For this review, take the finished solid that the model builds, in its own axes (mm). Round coordinates to 2 decimals unless told otherwise and drop trailing zeros. Order: outer loops, then holes, each group sorted by start corner. A loop starts at its lowest first (then second) coordinate and runs counter-clockwise, first axis right, second up. Notation, with made-up numbers: M -31,-33.75 L 20,-33.75 A4 ccw 20,-29.75 Z; hole C 15,-30 d8. An arc over 180 degrees is marked long. Use a Markdown table: item, result.
from build123d import *

# Parameters (mm, degrees)
BOSS_EXTRUDE1_DEPTH = 5
CHAMFER1_SIZE       = 3
SKETCH4_W           = 10
SKETCH4_H           = 2
BOSS_EXTRUDE3_DEPTH = 2
SKETCH5_W           = 2
SKETCH5_H           = 10
BOSS_EXTRUDE4_DEPTH = 12
CHAMFER2_SIZE       = 2
SKETCH6_W           = 10
SKETCH6_H           = 2
BOSS_EXTRUDE5_DEPTH = 1
CHAMFER3_SIZE       = 1
SKETCH7_W           = 10
SKETCH7_H           = 2
BOSS_EXTRUDE6_DEPTH = 2
SKETCH8_W           = 2
SKETCH8_H           = 10
BOSS_EXTRUDE7_DEPTH = 12
CHAMFER4_SIZE       = 2
SKETCH9_W           = 10
SKETCH9_H           = 2
BOSS_EXTRUDE8_DEPTH = 1
CHAMFER5_SIZE       = 1


with BuildPart() as part:
    # Sketch1 → Boss-Extrude1 (new body)
    with BuildSketch(Plane(origin=(0, 0, 0), x_dir=(1, 0, 0), z_dir=(0, 1, 0))):
        Polygon((-96.805555556, 26.527777778), (-46.805555556, 26.527777778), (-46.805555556, 76.527777778), (57.194444444, 76.527777778), (57.194444444, 26.527777778), (107.194444444, 26.527777778), (107.194444444, -43.472222222), (-96.805555556, -43.472222222), align=None)
    extrude(amount=BOSS_EXTRUDE1_DEPTH)

    # Chamfer1
    chamfer1_edges = [part.edges().sort_by_distance(p)[0] for p in [
        (107.194444444, 5, 8.472222222),
        (82.194444444, 5, -26.527777778),
        (57.194444444, 5, -51.527777778),
        (5.194444444, 5, -76.527777778),
        (-46.805555556, 5, -51.527777778),
        (-71.805555556, 5, -26.527777778),
        (-96.805555556, 5, 8.472222222),
        (5.194444444, 5, 43.472222222),
    ]]
    chamfer(chamfer1_edges, length=CHAMFER1_SIZE)

    # Sketch4 → Boss-Extrude3 (add)
    with BuildSketch(Plane(origin=(107.194444444, 0, 0), x_dir=(0, 0, -1), z_dir=(1, 0, 0))):
        with Locations((-8.472222222, 1)):
            Rectangle(SKETCH4_W, SKETCH4_H)
    extrude(amount=BOSS_EXTRUDE3_DEPTH)

    # Sketch5 → Boss-Extrude4 (add)
    with BuildSketch(Plane(origin=(0, 2, 0), x_dir=(1, 0, 0), z_dir=(0, 1, 0))):
        with Locations((108.194444444, -8.472222222)):
            Rectangle(SKETCH5_W, SKETCH5_H)
    extrude(amount=BOSS_EXTRUDE4_DEPTH)

    # Chamfer2
    chamfer2_edges = [part.edges().sort_by_distance(p)[0] for p in [
        (107.194444444, 14, 8.472222222),
    ]]
    chamfer(chamfer2_edges, length=CHAMFER2_SIZE - 0.0001)  # a hair under: the kernel refuses the full size

    # Sketch6 → Boss-Extrude5 (add)
    with BuildSketch(Plane.ZY.offset(-107.194444444)):
        with Locations((8.472222222, 11)):
            Rectangle(SKETCH6_W, SKETCH6_H)
    extrude(amount=BOSS_EXTRUDE5_DEPTH)

    # Chamfer3
    chamfer3_edges = [part.edges().sort_by_distance(p)[0] for p in [
        (106.194444444, 10, 8.472222222),
        (106.194444444, 12, 8.472222222),
    ]]
    chamfer(chamfer3_edges, length=CHAMFER3_SIZE - 0.0001)  # a hair under: the kernel refuses the full size

    # Sketch7 → Boss-Extrude6 (add)
    with BuildSketch(Plane.ZY.offset(96.805555556)):
        with Locations((8.472222222, 1)):
            Rectangle(SKETCH7_W, SKETCH7_H)
    extrude(amount=BOSS_EXTRUDE6_DEPTH)

    # Sketch8 → Boss-Extrude7 (add)
    with BuildSketch(Plane(origin=(0, 2, 0), x_dir=(1, 0, 0), z_dir=(0, 1, 0))):
        with Locations((-97.805555556, -8.472222222)):
            Rectangle(SKETCH8_W, SKETCH8_H)
    extrude(amount=BOSS_EXTRUDE7_DEPTH)

    # Chamfer4
    chamfer4_edges = [part.edges().sort_by_distance(p)[0] for p in [
        (-96.805555556, 14, 8.472222222),
    ]]
    chamfer(chamfer4_edges, length=CHAMFER4_SIZE - 0.0001)  # a hair under: the kernel refuses the full size

    # Sketch9 → Boss-Extrude8 (add)
    with BuildSketch(Plane(origin=(-96.805555556, 0, 0), x_dir=(0, 0, -1), z_dir=(1, 0, 0))):
        with Locations((-8.472222222, 11)):
            Rectangle(SKETCH9_W, SKETCH9_H)
    extrude(amount=BOSS_EXTRUDE8_DEPTH)

    # Chamfer5
    chamfer5_edges = [part.edges().sort_by_distance(p)[0] for p in [
        (-95.805555556, 10, 8.472222222),
        (-95.805555556, 12, 8.472222222),
    ]]
    chamfer(chamfer5_edges, length=CHAMFER5_SIZE - 0.0001)  # a hair under: the kernel refuses the full size


solid = part.part
Q1. Add section A-A (x = -7). Write out the cut boundary in (y, z).
Determined:
| item | result |
|---|---|
| outline | M 0,-76.53 L 2,-76.53 L 5,-73.53 L 5,40.47 L 2,43.47 L 0,43.47 Z |
Q2. Clearance check with flat-ended pins moving along their axes: pin 1 (1.6 mm diameter, centred on y = 0.5, z = 29, fed in from +X); pin 2 (0.9 mm diameter, centred on x = -97, y = 5, fed in from -Z); pin 3 (0.9 mm diameter, centred on x = 107, y = 6.5, fed in from +Z). State where each tip first meets the part, or that it passes through.
Determined:
| item | result |
|---|---|
| pin 1 | stops at x = 107.19 |
| pin 2 | stops at z = 3.47 |
| pin 3 | stops at z = 13.47 |
Q3. Wall thickness on line 1 along X through (y, z) = (6, 4.5); line 2 along Y through (x, z) = (4.5, -35); line 3 along X through (y, z) = (4, 10): over which ranges is each line inside the solid? List them lowest first. Write a range as [from, to].
Determined:
| item | result |
|---|---|
| line 1 | x = [-98.81, -96.81], [107.19, 109.19] |
| line 2 | y = [0, 5] |
| line 3 | x = [-98.81, -96.81], [-94.81, 105.19], [107.19, 109.19] |
Q4. Draft analysis for pull direction Y (two halves, no side actions). For faces 1 (the flat face through (-96.806, 6, 9)), 2 (the flat face through (7, 5, -5)), 3 (the flat face through (109.194, 7, 9)), state which applies: pulls with the +Y half, pulls with the -Y half, needs draft (parallel to the pull), parting line crosses it, or undercut.
Determined:
| item | result |
|---|---|
| face 1 | undercut |
| face 2 | pulls with the +Y half |
| face 3 | needs draft |
Q5. Add section B-B (z = -17). Write out the cut boundary in (x, y), then the cut area to 3 significant figures.
Determined:
| item | result |
|---|---|
| outline | M -96.81,0 L 107.19,0 L 107.19,2 L 104.19,5 L -93.81,5 L -96.81,2 Z |
| area | 1,010 mm^2 |
